Autodesk Inventor part; units mm, degrees
ref_plane "Arbeitsebene1" through (-9.7716, -9.2098, 6) normal (0, 0, 1) x (1, 0, 0)
ref_plane "YZ Plane" through (0, 0, 0) normal (1, 0, 0) x (0, 1, 0)
ref_plane "XZ Plane" through (0, 0, 0) normal (0, 1, 0) x (-1, 0, 0)
sketch "Skizze1" plane through (0, 0, 0) normal (0, 0, 1) x (1, 0, 0)
  line L0 (14.1792, -17.284) -> (14.1792, 17.716)
  line L1 (14.1792, 17.716) -> (-11.8208, 17.716)
  line L2 (-11.8208, 17.716) -> (-11.8208, -17.284)
  line L3 (-11.8208, -17.284) -> (14.1792, -17.284)
  line L4 (14.1792, -17.284) -> (-11.8208, 17.716) construction
  line L5 (14.1792, 17.716) -> (-11.8208, -17.284) construction
  line L6 (3.4292, 10.341) -> (-6.0708, 10.341) construction
  line L7 (3.4292, 3.091) -> (3.4292, 10.341) construction
  line L8 (-6.0708, 3.091) -> (3.4292, 3.091) construction
  line L9 (-6.0708, 10.341) -> (-6.0708, 3.091) construction
  line L10 (3.4292, 10.341) -> (-6.0708, 3.091) construction
  line L11 (3.4292, 3.091) -> (-6.0708, 10.341) construction
  point P0 (0, 0)
  point P1 (1.1792, 0.216)
  point P2 (1.1792, 0.216)
  point P3 (-1.3208, 6.716)
  point P4 (-1.3208, 6.716)
  point P5 (1.1792, 0.216)
  point P6 (-1.3208, 6.716)
  dimension "d0" = 26
  dimension "d1" = 35
  dimension "d2" = 11
  dimension "d3" = 2.5
sketch "Skizze2" plane through (0, 0, 0) normal (0, 0, 1) x (1, 0, 0)
  line L0 (-3.4208, 1.091) -> (-7.8208, 1.091)
  line L1 (-7.8208, 1.091) -> (-7.8208, 12.341)
  line L2 (-7.8208, 12.341) -> (-3.4208, 12.341)
  line L3 (5.1792, 1.091) -> (0.7792, 1.091)
  line L4 (5.1792, 12.341) -> (5.1792, 1.091)
  line L5 (0.7792, 12.341) -> (5.1792, 12.341)
  circle A0 centre (-9.3002, -4.7384) radius 1.575 construction
  circle A1 centre (11.3792, 14.191) radius 1.575 construction
  circle A2 centre (-9.3002, -4.7384) radius 0.7 construction
  circle A3 centre (-10.7708, 16.016) radius 0.7 construction
  circle A4 centre (11.3792, 14.191) radius 0.7 construction
  line L6 (-3.4208, 12.341) -> (-3.4208, 13.366)
  line L7 (-3.4208, 13.366) -> (0.7792, 13.366)
  line L8 (0.7792, 0.066) -> (-3.4208, 0.066)
  line L9 (-3.4208, 0.066) -> (-3.4208, 1.091)
  line L10 (0.7792, 1.091) -> (0.7792, 0.066)
  line L11 (0.7792, 13.366) -> (0.7792, 12.341)
  line L12 (-12.2708, -9.259) -> (-12.2708, 10.741) construction
  line L13 (14.5292, 16.566) -> (-9.295, 16.566) construction
  arc A5 (16.5292, 14.566) -> (14.5292, 16.566) centre (14.5292, 14.566) ccw
  line L14 (16.5292, 14.566) -> (16.5292, 13.191)
  arc A6 (15.5292, 12.191) -> (16.5292, 13.191) centre (15.5292, 13.191) ccw
  line L15 (15.5292, 12.191) -> (14.4292, 12.191)
  arc A7 (14.4292, 12.191) -> (12.4292, 10.191) centre (14.4292, 10.191) ccw
  line L16 (12.4292, 10.191) -> (12.4292, -3.209)
  line L17 (-3.5708, -3.209) -> (12.4292, -3.209)
  line L18 (-8.1002, -7.7384) -> (-3.5708, -3.209)
  arc A8 (-10.7708, 17.591) -> (-9.295, 16.566) centre (-10.7708, 16.016) ccw construction
  line L19 (-8.1002, -8.7384) -> (-8.1002, -7.7384) construction
  circle A9 centre (-9.3002, -8.7384) radius 0.75 construction
  circle A10 centre (-9.3002, -8.7384) radius 1.2 construction
  line L20 (-10.8208, -7.909) -> (-11.8208, -6.909) construction
  line L21 (-11.8208, -6.909) -> (-11.8208, 14.7109)
  line L22 (-11.8208, -6.909) -> (-10.4976, -8.2322)
  arc A11 (-8.1002, -8.2384) -> (-8.2864, -7.9246) centre (-9.3002, -8.7384) ccw construction
  line L23 (-8.1002, -8.2384) -> (-8.1002, -7.7384) construction
  circle A12 centre (-9.3002, -4.7384) radius 1.675
  circle A13 centre (11.3792, 14.191) radius 1.675
  line L24 (14.5292, 16.566) -> (-9.1887, 16.566)
  arc A14 (-11.8208, 14.7109) -> (-9.1887, 16.566) centre (-10.7708, 16.016) ccw
  circle A15 centre (14.3792, 14.191) radius 0.75 construction
  circle A16 centre (14.3792, 14.191) radius 0.85
  line L25 (-8.1002, -7.7384) -> (-8.2864, -7.9246)
  arc A17 (-8.2864, -7.9246) -> (-10.4976, -8.2322) centre (-9.3002, -8.7384) ccw
  point P0 (0, 0)
  dimension "d4" = 0.1
  dimension "d5" = 0.1
  dimension "d6" = 0.1
  dimension "d7" = 0.1
  dimension "d10" = 0.1
extrude "Extrusion1" add sketch "Skizze2" along normal blind 2.5
sketch "Skizze3" plane through (0, 0, 2.5) normal (0, 0, 1) x (1, 0, 0)
  line L0 (-7.8208, 1.091) -> (-7.8208, 12.341)
  line L1 (-7.8208, 12.341) -> (-3.4208, 12.341)
  line L2 (-3.4208, 12.341) -> (-3.4208, 13.366)
  line L3 (-3.4208, 13.366) -> (0.7792, 13.366)
  line L4 (0.7792, 13.366) -> (0.7792, 12.341)
  line L5 (0.7792, 12.341) -> (5.1792, 12.341)
  line L6 (5.1792, 12.341) -> (5.1792, 1.091)
  line L7 (5.1792, 1.091) -> (0.7792, 1.091)
  line L8 (0.7792, 1.091) -> (0.7792, 0.066)
  line L9 (0.7792, 0.066) -> (-3.4208, 0.066)
  line L10 (-3.4208, 0.066) -> (-3.4208, 1.091)
  line L11 (-3.4208, 1.091) -> (-7.8208, 1.091)
  circle A0 centre (11.3792, 14.191) radius 1.675 construction
  circle A1 centre (-9.3002, -4.7384) radius 1.675 construction
  circle A2 centre (14.3792, 14.191) radius 0.85
  arc A3 (16.5292, 14.566) -> (14.5292, 16.566) centre (14.5292, 14.566) ccw
  line L12 (14.5292, 16.566) -> (-9.1887, 16.566)
  arc A4 (-11.8208, 14.7109) -> (-9.1887, 16.566) centre (-10.7708, 16.016) ccw construction
  line L13 (-11.8208, 14.7109) -> (-11.8208, -6.909)
  line L14 (-11.8208, -6.909) -> (-10.4976, -8.2322)
  line L15 (-8.2864, -7.9246) -> (-3.5708, -3.209)
  line L16 (-3.5708, -3.209) -> (12.4292, -3.209)
  line L17 (12.4292, -3.209) -> (12.4292, 10.191)
  arc A5 (14.4292, 12.191) -> (12.4292, 10.191) centre (14.4292, 10.191) ccw
  line L18 (14.4292, 12.191) -> (15.5292, 12.191)
  arc A6 (15.5292, 12.191) -> (16.5292, 13.191) centre (15.5292, 13.191) ccw
  line L19 (16.5292, 13.191) -> (16.5292, 14.566)
  circle A7 centre (11.3792, 14.191) radius 0.7 construction
  circle A8 centre (-9.3002, -4.7384) radius 0.7 construction
  circle A9 centre (-9.3002, -8.7384) radius 0.75 construction
  arc A10 (-8.2864, -7.9246) -> (-10.4976, -8.2322) centre (-9.3002, -8.7384) ccw construction
  circle A11 centre (-9.3002, -8.7384) radius 0.85
  line L20 (-8.2864, -7.9246) -> (-3.5708, -3.209)
  arc A12 (-10.4976, -8.2322) -> (-8.2864, -7.9246) centre (-9.3002, -8.7384) ccw
  arc A13 (-9.1887, 16.566) -> (-11.8208, 14.7109) centre (-10.7708, 16.016) ccw
  circle A14 centre (-10.7708, 16.016) radius 0.7 construction
  circle A15 centre (-10.7708, 16.016) radius 0.9
  circle A16 centre (11.3792, 14.191) radius 0.9
  circle A17 centre (-9.3002, -4.7384) radius 0.9
  point P0 (0, 0)
  dimension "d11" = 0.1
  dimension "d13" = 1.8
  dimension "d14" = 1.8
  dimension "d15" = 1.8
ref_plane "Arbeitsebene1" through (-9.7716, -9.2098, 6) normal (0, 0, 1) x (1, 0, 0)
extrude "Extrusion2" add sketch "Skizze3" along normal up to surface (3.5 mm away) contours L19 A6 L18 A5 L17 L16 L15 A12 L14 L13 A13 L12 A3 | A16 | A17
sketch "Skizze4" plane through (-9.1887, 16.566, 6) normal (0, 0, 1) x (1, 0, 0)
  circle A0 centre (-0.1115, -21.3043) radius 0.7 construction
  circle A1 centre (-1.5821, -0.55) radius 0.7 construction
  circle A2 centre (20.5679, -2.375) radius 0.7 construction
  point P0 (9.1887, -16.566)
hole "Bohrung1" at (-9.3002, -4.7384, 6) at (11.3792, 14.191, 6) direction (0, 0, -1) diameter 1.8 end through all counterbore diameter 3.5 counterbore depth 1.8
sketch "Sketch5" plane through (-9.1887, 16.566, 6) normal (0, 0, 1) x (1, 0, 0)
  circle A0 centre (7.7527, -12.1874) radius 3.65
  circle A1 centre (-0.1115, -21.3043) radius 1.75
  circle A2 centre (20.5679, -2.375) radius 1.75
  line L0 (25.7179, -2) -> (25.7179, -3.375)
  arc A3 (25.7179, -2) -> (23.7179, 0) centre (23.7179, -2) ccw
  line L1 (0, 0) -> (23.7179, 0)
  arc A4 (0, 0) -> (-2.6321, -1.855) centre (-1.5821, -0.55) ccw
  line L2 (-2.6321, -23.475) -> (-2.6321, -1.855)
  line L3 (-1.3089, -24.7982) -> (-2.6321, -23.475)
  arc A5 (-1.3089, -24.7982) -> (0.9023, -24.4906) centre (-0.1115, -25.3043) ccw
  line L4 (5.6179, -19.775) -> (0.9023, -24.4906)
  line L5 (21.6179, -19.775) -> (5.6179, -19.775)
  line L6 (21.6179, -6.375) -> (21.6179, -19.775)
  arc A6 (23.6179, -4.375) -> (21.6179, -6.375) centre (23.6179, -6.375) ccw
  line L7 (24.7179, -4.375) -> (23.6179, -4.375)
  arc A7 (24.7179, -4.375) -> (25.7179, -3.375) centre (24.7179, -3.375) ccw
  circle A8 centre (23.5679, -2.375) radius 0.85
  circle A9 centre (-0.1115, -25.3043) radius 0.85
  circle A10 centre (-1.5821, -0.55) radius 0.9
  line L8 (5.7679, -4.225) -> (1.3679, -4.225)
  line L9 (5.7679, -3.2) -> (5.7679, -4.225)
  line L10 (9.9679, -3.2) -> (5.7679, -3.2)
  line L11 (9.9679, -4.225) -> (9.9679, -3.2)
  line L12 (14.3679, -4.225) -> (9.9679, -4.225)
  line L13 (14.3679, -15.475) -> (14.3679, -4.225)
  line L14 (9.9679, -15.475) -> (14.3679, -15.475)
  line L15 (9.9679, -16.5) -> (9.9679, -15.475)
  line L16 (5.7679, -16.5) -> (9.9679, -16.5)
  line L17 (5.7679, -15.475) -> (5.7679, -16.5)
  line L18 (1.3679, -15.475) -> (5.7679, -15.475)
  line L19 (1.3679, -4.225) -> (1.3679, -15.475)
  point P0 (9.1887, -16.566)
  dimension "d25" = 7.3
extrude "Extrusion3" add sketch "Sketch5" against normal up to surface (6 mm away) contours L9 L10 L11 L12 L13 L14 L15 L16 L17 L18 L19 L8
sketch "Sketch6" plane through (12.4292, -3.209, 0) normal (1, 0, 0) x (0, 0, -1)
  line L0 (0, 13.4) -> (0, 0)
  line L1 (0, 13.4) -> (-6, 13.4)
  line L2 (-6, 13.4) -> (-6, 0)
  line L3 (0, 0) -> (-6, 0)
  circle A0 centre (-3, 6.4105) radius 1.45
  point P0 (0, 3.209)
  dimension "d28" = 2.9
extrude "Extrusion4" cut sketch "Sketch6" against normal through all contours A0
properties part number "110_Syrringeholder_XY_Stage"
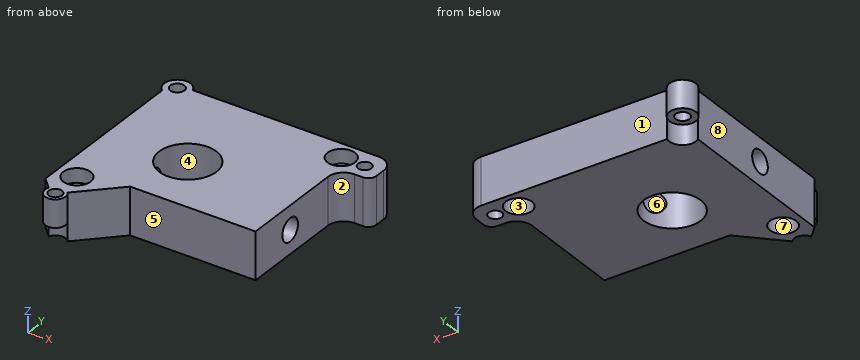
The listing builds one solid part. Answer for the finished solid, in the listing's coordinates (mm). Face numbers are marked on the shaded views. A direction names the side the tool comes from. Round coordinates to 2 decimals unless told otherwise and drop trailing zeros. Order: outer loops, then holes, each group sorted by start corner. A loop starts at its lowest first (then second) coordinate and runs counter-clockwise, first axis right, second up. Notation, with made-up numbers: (25.25, 34.5) -> (52.25, 34.5) arc R18 ccw to (52.25, 62.5) -> close; hole circle Ø11 at (57, 7.25). An arc over 180 degrees is marked (long way). One line per item, written item: value.
Item 1: Find section D-D, the plane z = 5.5. Give the vertices of the cut face in (x, y) (3 decimals), then the cut area to 3 significant figures.
Taken from the geometry:
outline: (-11.821, -6.909) -> (-10.498, -8.232) arc R1.3 ccw (long way) to (-8.286, -7.925) -> (-3.571, -3.209) -> (12.429, -3.209) -> (12.429, 10.191) arc R2 cw to (14.429, 12.191) -> (15.529, 12.191) arc R1 ccw to (16.529, 13.191) -> (16.529, 14.566) arc R2 ccw to (14.529, 16.566) -> (-9.189, 16.566) arc R1.675 ccw (long way) to (-11.821, 14.711) -> close; hole circle Ø1.8 at (-10.771, 16.016); hole circle Ø3.5 at (-9.3, -4.738); hole circle Ø1.7 at (-9.3, -8.738); hole circle Ø7.3 at (-1.436, 4.379); hole circle Ø3.5 at (11.379, 14.191); hole circle Ø1.7 at (14.379, 14.191)
area: 465 mm2
Item 2: Find section A-A, the plane z = 3. State how many separate pieces and enclosed holes the cut face has, then the cut area to 3 significant figures.
Taken from the geometry:
separate pieces: 2
enclosed holes: 5
area: 428 mm2
Item 3: Given P1, Ø1.8, axis at x = 5.5, z = 4, coming from the +Y side; P2, Ø1.7, axis at x = -9.5, y = -5, coming from the -Z side; P3, Ø1.5, axis at x = 9.5, z = 2, coming from the -Y side, each flat-ended and moving along its own axis, determine where each tip first touches the part or whether it passes through.
Taken from the geometry:
P1: stops at y = 16.57
P2: stops at z = 2.5
P3: stops at y = -3.21
Item 4: Straight lines are drawn through the part: L1, parallel to Y at x = -1.25, z = 4.75; L2, parallel to Y at x = -9.25, z = 2.25; L3, parallel to X at y = 13.5, z = 4.75. For each, find the intervals that lie inside material, in ascending order.
Taken from the geometry:
L1: y = -3.21 to 0.73, 8.02 to 16.57
L2: y = -7.44 to -6.41, -3.06 to 1.96, 4.44 to 15.31
L3: x = -11.82 to 9.77, 12.99 to 13.88, 14.87 to 16.53
Item 5: For the marked faces 4, 5, 6, 7 and 8, determine the directions among +Z, -Z, +X, -X, +Y, -Y from which every point of the face is accessible in a straight line to the end or side of a thin tool.
Taken from the geometry:
face 4: +Z, -Z
face 5: +Z, -Z, +X, -Y
face 6: +X, -X
face 7: -Z
face 8: +Z, -Z, -X, -Y
Item 6: Find section C-C, the plane z = 1. Give the vertices of the cut face in (x, y) (3 decimals).
Taken from the geometry:
outline: (-11.821, -6.909) -> (-10.498, -8.232) arc R1.3 cw to (-8.286, -7.925) -> (-3.571, -3.209) -> (12.429, -3.209) -> (12.429, 10.191) arc R2 cw to (14.429, 12.191) -> (15.529, 12.191) arc R1 ccw to (16.529, 13.191) -> (16.529, 14.566) arc R2 ccw to (14.529, 16.566) -> (-9.189, 16.566) arc R1.675 cw to (-11.821, 14.711) -> close; hole circle Ø3.35 at (-9.3, -4.738); hole circle Ø7.3 at (-1.436, 4.379); hole circle Ø3.35 at (11.379, 14.191); hole circle Ø1.7 at (14.379, 14.191)
Item 7: For a pull along X with two mould halves and no side action, classify the marked faces 1, 2 and 3 as released by +X, released by -X, zero draft, split by the parting line, or undercut.
Taken from the geometry:
face 1: zero draft
face 2: released by +X
face 3: undercut
Item 8: Find section B-B, the plane x = 6. Give the vertices of the cut face in (y, z), then the cut area to 3 significant figures.
Taken from the geometry:
outline: (-3.21, 0) -> (16.57, 0) -> (16.57, 6) -> (-3.21, 6) -> close; hole circle Ø2.9 at (3.2, 3)
area: 112 mm2
